```python
from build123d import *

# Parameters (mm, degrees)
EXTRUDE_1_DEPTH     = 2
SKETCH_2_R          = 4.5
SKETCH_2_R_2        = 1.5
CUT_EXTRUDE_1_DEPTH = 2


with BuildPart() as part:
    # 草图1 → 凸台-拉伸1 (new body)
    with BuildSketch(Plane.XY):
        with BuildLine():
            ThreePointArc((-27.528089888, 5.866903721), (-41.670339741, 6.764360114), (-40.970905632, -7.389065295))
            ThreePointArc((-40.970905632, -7.389065295), (0, -21.87378703), (40.970905632, -7.389065295))
            ThreePointArc((40.970905632, -7.389065295), (41.670339741, 6.764360114), (27.528089888, 5.866903721))
            ThreePointArc((27.528089888, 5.866903721), (0, -7.518187833), (-27.528089888, 5.866903721))
        make_face()
    extrude(amount=EXTRUDE_1_DEPTH)

    # 草图2 → 切除-拉伸1 (cut)
    with BuildSketch(Plane.XY.offset(2)):
        with Locations((35, 0)):
            Circle(SKETCH_2_R)
        with Locations((-35, 0)):
            Circle(SKETCH_2_R)
        with Locations((-28, 0)):
            Circle(SKETCH_2_R_2)
        with Locations((-35, -7)):
            Circle(SKETCH_2_R_2)
        with Locations((-42, 0)):
            Circle(SKETCH_2_R_2)
        with Locations((-35, 7)):
            Circle(SKETCH_2_R_2)
        with Locations((28, 0)):
            Circle(SKETCH_2_R_2)
        with Locations((35, 7)):
            Circle(SKETCH_2_R_2)
        with Locations((42, 0)):
            Circle(SKETCH_2_R_2)
        with Locations((35, -7)):
            Circle(SKETCH_2_R_2)
    extrude(amount=-CUT_EXTRUDE_1_DEPTH, mode=Mode.SUBTRACT)


solid = part.part
```
The model under review builds one solid part; all positions refer to its coordinate system, in mm. Round coordinates to 2 decimals unless told otherwise and drop trailing zeros. Write each loop counter-clockwise with the first axis right and the second up, starting at its lowest first coordinate (ties: lowest second). Pieces come first, ordered by that corner, then holes.
(1) We need section A-A on z = 0.3. Give the number of separate pieces and of enclosed holes in the cut face, and give its area (3 significant figures).
(2) We need section B-B on x = -35. Give the boundary of the cut face in (y, z).
(3) We need section C-C on y = 7. Give the boundary of the cut face in (x, z), and give its area (3 significant figures).
(4) Mouldability with a two-part tool opening along X and no side actions: class faces 1 (the flat face through (-1, -9, 0)), 2 (the cylindrical face through (-43.5, 0.07, 1.01)), 3 (the cylindrical face through (-36.2, 6.1, 1)), 4 (the cylindrical face through (-0.62, -21.87, 0.99)) as +X half, -X half, draft (parallel to the pull), parting line (faces both ways), or undercut.
(5) Wall thickness on L1, parallel to Y at x = 34, z = 1.4; L2, parallel to X at y = -4, z = 1.05; L3, parallel to Y at x = 35, z = 0.95: over which ranges is each line inside the solid? List them lowest first.
(6) Insertion check: pin 1 (2.5 mm diameter, centred on x = 35, y = 7, fed in from +Z); pin 2 (1 mm diameter, centred on y = 3.5, z = 0.5, fed in from +X). Each pin has a flat end and moves straight along its axis. Give the tip position at first contact, or say it passes through.
(7) We need section D-D on x = 42. Give the boundary of the cut face in (y, z), and give its area (3 significant figures).
Findings below:
1. separate pieces: 1
1. enclosed holes: 10
1. area: 1,350 mm2
2. outline: (-11.68, 0) - (-8.5, 0) - (-8.5, 2) - (-11.68, 2) - close; (-5.5, 0) - (-4.5, 0) - (-4.5, 2) - (-5.5, 2) - close; (4.5, 0) - (5.5, 0) - (5.5, 2) - (4.5, 2) - close; (8.5, 0) - (9.5, 0) - (9.5, 2) - (8.5, 2) - close
3. outline: (-41.42, 0) - (-36.5, 0) - (-36.5, 2) - (-41.42, 2) - close; (-33.5, 0) - (-28.58, 0) - (-28.58, 2) - (-33.5, 2) - close; (28.58, 0) - (33.5, 0) - (33.5, 2) - (28.58, 2) - close; (36.5, 0) - (41.42, 0) - (41.42, 2) - (36.5, 2) - close
3. area: 39.4 mm2
4. face 1: draft
4. face 2: undercut
4. face 3: undercut
4. face 4: parting line
5. L1: y = -12.3 to -8.12, -5.88 to -4.39, 4.39 to 5.88, 8.12 to 9.45
5. L2: x = -43.62 to -37.06, -32.94 to -15.29, 15.29 to 32.94, 37.06 to 43.62
5. L3: y = -11.68 to -8.5, -5.5 to -4.5, 4.5 to 5.5, 8.5 to 9.5
6. pin 1: passes through
6. pin 2: stops at x = 44.01
7. outline: (-6.42, 0) - (-1.5, 0) - (-1.5, 2) - (-6.42, 2) - close; (1.5, 0) - (6.42, 0) - (6.42, 2) - (1.5, 2) - close
7. area: 19.7 mm2
